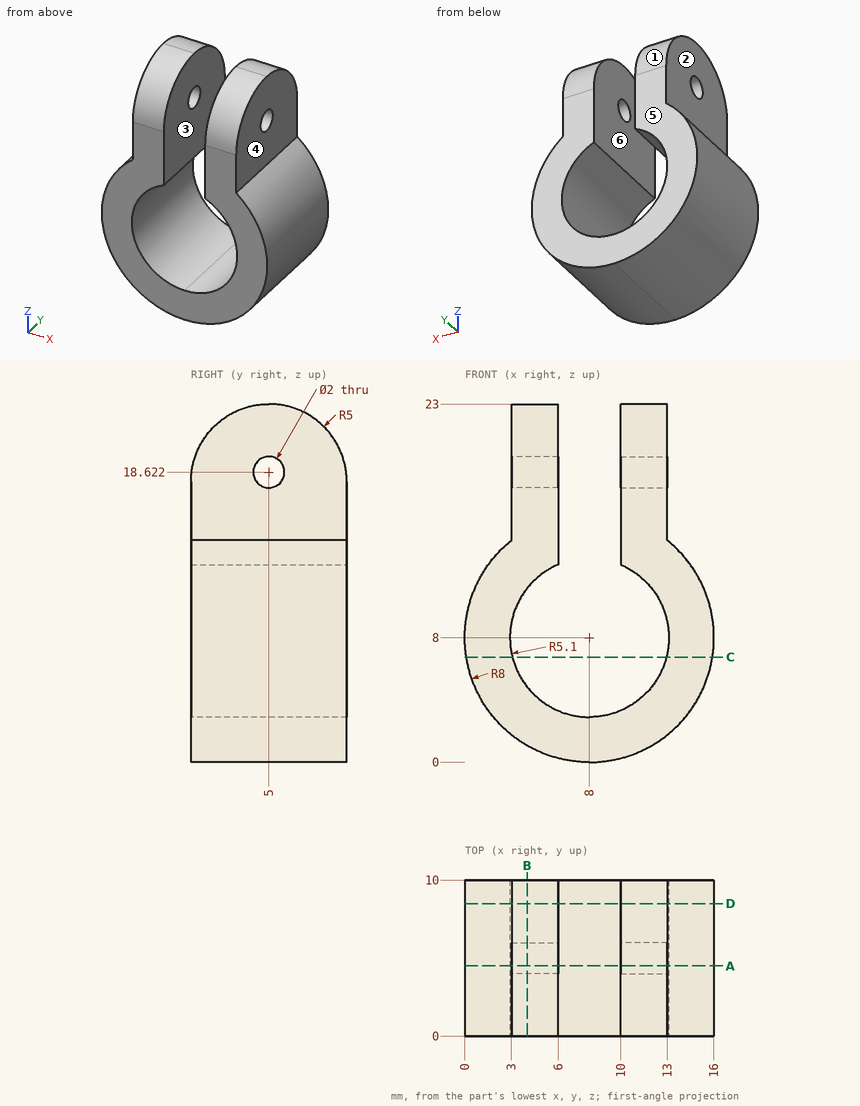
The drawing under review shows one solid part. Ordinate dimensions are in mm from its lowest x, y, z. A direction names the side the tool comes from. Coordinates: 2 decimals unless noted, no trailing zeros. Order: outer loops, then holes, each group sorted by start corner. A loop starts at its lowest first (then second) coordinate and runs counter-clockwise, first axis right, second up. Notation, with made-up numbers: (26.5, 47) -> (37.5, 47) arc R23 ccw to (37.5, 71) -> close; hole circle Ø8 at (60.5, 74.25). An arc over 180 degrees is marked (long way). Answer as CSV lines item,"result".
Q1. We need section B-B (x = 4). Count the separate pieces of the cut face and the enclosed holes in it, plus the area to 3 significant figures.
Model answer:
separate pieces,"2"
enclosed holes,"1"
area,"142 mm2"
Q2. Clearance check with flat-ended pins moving along their axes: pin 1 Ø4 at (y, z) = (3, 18.5) entering from +X; pin 2 Ø2 at (y, z) = (7, 19.5) entering from -X; pin 3 Ø1 at (x, y) = (10, 4) entering from -Z. State where each tip first meets the part, or that it passes through.
Model answer:
pin 1,"stops at x = 13"
pin 2,"stops at x = 3"
pin 3,"stops at z = 0.14"
Q3. We need section C-C (z = 6.75). State the section outline as (x, y) points (1 decimal).
Model answer:
outline,"(0.1, 0) -> (3.1, 0) -> (3.1, 10) -> (0.1, 10) -> close; (12.9, 0) -> (15.9, 0) -> (15.9, 10) -> (12.9, 10) -> close"
Q4. Wall thickness on line 1 along X through (y, z) = (1.25, 15); line 2 along Z through (x, y) = (4.8, 5) (1 decimal); line 3 along Z through (x, y) = (4.5, 5) (1 decimal): over which ranges is each line inside the solid? List them lowest first. Write a range as [from, to].
Model answer:
line 1,"x = [3, 6], [10, 13]"
line 2,"z = [0.7, 4], [12, 17.6], [19.6, 23]"
line 3,"z = [0.8, 4.3], [11.7, 17.6], [19.6, 23]"
Q5. For the marked faces 5 and 6, list the 3-axis set-ups (+Z, -Z, +X, -X, +Y, -Y) from which the entire face can be reached by the end or side of a thin tool; tool diameter is ignored.
Model answer:
face 5,"+Z, -Z, +X, -X, +Y"
face 6,"+Z, +Y, -Y"
Q6. Draft analysis for pull direction X (two halves, no side actions). For the marked faces 1, 2, 3 and 4, state which applies: released by +X, released by -X, zero draft, split by the parting line, or undercut.
Model answer:
face 1,"zero draft"
face 2,"released by -X"
face 3,"undercut"
face 4,"released by +X"
Q7. We need section D-D (y = 8.5). State the section outline as (x, z) points (1 decimal), plus the area to 3 significant figures.
Model answer:
outline,"(3, 14.2) arc R8 ccw (long way) to (13, 14.2) -> (13, 21.6) -> (10, 21.6) -> (10, 12.7) arc R5.1 cw (long way) to (6, 12.7) -> (6, 21.6) -> (3, 21.6) -> close"
area,"146 mm2"
Q8. We need section A-A (y = 4.5). State the section outline as (x, z) points (1 decimal), plus the area to 3 significant figures.
Model answer:
outline,"(3, 14.2) arc R8 ccw (long way) to (13, 14.2) -> (13, 17.8) -> (10, 17.8) -> (10, 12.7) arc R5.1 cw (long way) to (6, 12.7) -> (6, 17.8) -> (3, 17.8) -> close; (3, 19.5) -> (6, 19.5) -> (6, 23) -> (3, 23) -> close; (10, 19.5) -> (13, 19.5) -> (13, 23) -> (10, 23) -> close"
area,"144 mm2"
